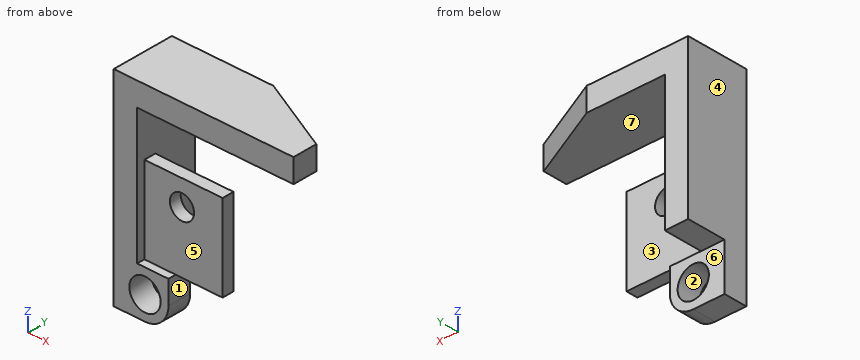
Autodesk Inventor part; units mm, degrees
ref_plane "YZ Plane" through (0, 0, 0) normal (1, 0, 0) x (0, 1, 0)
ref_plane "XZ Plane" through (0, 0, 0) normal (0, 1, 0) x (-1, 0, 0)
ref_plane "XY Plane" through (0, 0, 0) normal (0, 0, 1) x (1, 0, 0)
sketch "Szkic1" plane through (0, 0, 0) normal (0, 1, 0) x (-1, 0, 0)
  line L0 (0, 0) -> (3, 0)
  line L1 (3, 0) -> (3, -22)
  line L2 (3, -22) -> (0, -22)
  line L3 (0, -22) -> (0, 0)
  line L4 (0, 0) -> (-20, 0)
  line L5 (-20, 0) -> (-20, -3)
  line L6 (-20, -3) -> (0, -3)
  line L7 (0, -3) -> (0, 0)
  line L8 (0, -22) -> (-3, -22)
  line L9 (-3, -22) -> (-3, -17)
  line L10 (-3, -17) -> (0, -17)
  line L11 (0, -17) -> (0, -22)
  dimension "d0" = 3
  dimension "d1" = 22
  dimension "d2" = 20
  dimension "d3" = 3
  dimension "d4" = 3
  dimension "d5" = 5
extrude "Wyciągnięcie proste1" add sketch "Szkic1" along normal blind 8
sketch "Szkic2" plane through (20, 0, -3) normal (0, 0, -1) x (-1, 0, 0)
  line L0 (0, 0) -> (0, 8)
  line L1 (0, 0) -> (20, 8)
  line L2 (23, 8) -> (0, 8)
  point P0 (20, 0)
extrude "Wyciągnięcie proste2" cut sketch "Szkic2" against normal blind 3
sketch "Szkic3" plane through (0, 8, 0) normal (0, 1, 0) x (1, 0, 0)
  point P0 (0, 0)
sketch "Szkic4" plane through (3, 0, -17) normal (1, 0, 0) x (0, 0, -1)
  line L0 (5, 0) -> (5, 8)
  line L1 (0, 0) -> (0, 8)
  line L2 (5, 0) -> (0, 0)
  line L3 (0, 0) -> (0, 8)
  line L4 (0, 8) -> (5, 8)
  line L5 (5, 8) -> (5, 0)
  point P0 (-17, 0)
extrude "Wyciągnięcie proste3" cut sketch "Szkic4" against normal blind 3
sketch "Szkic5" plane through (0, 0, -22) normal (0, 0, -1) x (-1, 0, 0)
  line L0 (3, 8) -> (0, 8)
  line L1 (0, 0) -> (3, 0)
  line L2 (3, 0) -> (3, 8)
  line L3 (3, 8) -> (0, 8)
  line L4 (0, 8) -> (0, 0)
extrude "Wyciągnięcie proste4" cut sketch "Szkic5" against normal blind 1.8
sketch "Szkic6" plane through (0, 0, -20.2) normal (0, 0, -1) x (-1, 0, 0)
  line L0 (3, 0) -> (3, 8)
  line L1 (3, 0) -> (-4, 0)
  line L2 (-4, 0) -> (-4, 3)
  line L3 (-4, 3) -> (3, 3)
  line L4 (3, 3) -> (3, 0)
  point P0 (0, 0)
  dimension "d14" = 7
  dimension "d15" = 3
extrude "Wyciągnięcie proste5" add sketch "Szkic6" along normal blind 6
sketch "Szkic7" plane through (0, 3, -20.2) normal (0, 1, 0) x (1, 0, 0)
  circle A0 centre (1, 3) radius 2
  line L0 (-3, 0) -> (-3, 6)
  line L1 (-3, 6) -> (4, 6)
  point P0 (0, -20.2)
  point P1 (-3, 3)
  point P2 (0.5, 6)
  dimension "d18" = 4
  dimension "d19" = 4
  dimension "d20" = 3
extrude "Wyciągnięcie proste6" cut sketch "Szkic7" against normal blind 3
sketch "Szkic8" plane through (-3, 0, 0) normal (0, 0, 1) x (1, 0, 0)
  line L0 (3, 8) -> (13, 8)
  line L1 (23, 0) -> (3, 0)
  line L2 (23, 0) -> (23, 3.137)
  line L3 (13, 8) -> (23, 3.137)
  line L4 (23, 0) -> (3, 8)
  line L5 (3, 8) -> (23, 0)
  dimension "d23" = 10
  dimension "d24" = 3.137
extrude "Wyciągnięcie proste7" add sketch "Szkic8" against normal blind 3
sketch "Szkic9" plane through (0, 0, -3) normal (1, 0, 0) x (0, 0, -1)
  line L0 (0, 0) -> (17.2, 0)
  line L1 (17.2, 0) -> (6.2, 0)
  line L2 (6.2, 0) -> (6.2, 1.5)
  line L3 (6.2, 1.5) -> (17.2, 1.5)
  line L4 (17.2, 1.5) -> (17.2, 0)
  point P0 (-3, 0)
  point P1 (6.2, 0)
  dimension "d27" = 11
  dimension "d35" = 1.5
extrude "Wyciągnięcie proste8" add sketch "Szkic9" along normal blind 10
sketch "Szkic10" plane through (0, 1.5, -9.2) normal (0, 1, 0) x (1, 0, 0)
  circle A0 centre (4.8, 3.2) radius 1.55
  line L0 (0, 0) -> (10, 0)
  line L1 (10, 11) -> (10, 0)
  line L2 (4, 11) -> (10, 11)
  line L3 (0, -6.2) -> (0, 11)
  point P0 (0, -9.2)
  point P1 (5, 0)
  dimension "d30" = 3.1
  dimension "d36" = 7.8
  dimension "d37" = 4.8
extrude "Wyciągnięcie proste9" cut sketch "Szkic10" against normal blind 2
fillet "Fillet1" radius 3 1 edges at (4, 1.5, -26.2)
sketch "Szkic11" plane through (0, 1.5, -9.2) normal (0, 1, 0) x (1, 0, 0)
  circle A0 centre (4.8, 3.2) radius 1.55
  line L0 (0, 0) -> (0, 11)
  line L1 (0, 0) -> (10, 0)
  line L2 (10, 11) -> (10, 0)
  line L3 (4, 11) -> (10, 11)
  line L4 (0, 11) -> (4, 11)
  point P0 (0, -9.2)
extrude "Wyciągnięcie proste10" add sketch "Szkic11" along normal blind 1
sketch "Szkic12" plane through (0, 0, 0) normal (0, -1, 0) x (1, 0, 0)
  line L0 (10, -9.2) -> (10, -20.2)
  line L1 (10, -20.2) -> (4, -20.2)
  line L2 (0, -20.2) -> (4, -20.2)
  line L3 (0, -9.2) -> (0, -20.2)
  line L4 (0, -9.2) -> (10, -9.2)
  circle A0 centre (4.8, -12.4) radius 1.55
  point P0 (0, 0)
extrude "Wyciągnięcie proste11" cut sketch "Szkic12" against normal blind 1
properties part number "lfmw" material "Tworzywo sztuczne PET"
The listing builds one solid part. Answer for the finished solid, in the listing's coordinates (mm). Face numbers are marked on the shaded views. A direction names the side the tool comes from. Round coordinates to 2 decimals unless told otherwise and drop trailing zeros. Loops run counter-clockwise (first coordinate to the right, second up) from the corner with the lowest first, then second, coordinate; pieces in that order, holes last. Notation, with made-up numbers: (33, 26.5) - (82, 26.5) arc R31 ccw to (82, 65.5) - close; hole circle Ø7 at (40, 65). An arc over 180 degrees is marked (long way). Return JSON: item names as keys, results as strings. Group by question number.
1. Which of the six approach directions +Z, -Z, +X, -X, +Y, -Y give full straight-line access (tool end or side, diameter ignored) to the marked faces 5, 6 and 7?
2. The part is cut by section A-A on x = 4.8. Determine the outline of the cut face in (y, z).
3. The part is cut by section D-D on z = -15.75. Determine the outline of the cut face in (x, y).
4. Each of these flat-tipped pins is pushed along its axis until it touches: P1, Ø2, axis at x = 6.5, z = -20, coming from the -Y side; P2, Ø3.5, axis at y = 1, z = -21, coming from the +X side; P3, Ø1, axis at x = 6, z = -14.5, coming from the +Y side; P4, Ø1, axis at x = 13, y = 1, coming from the +Z side. Where does it stop, or does it pass through?
5. The part is cut by section C-C on y = 2. Determine the outline of the cut face in (x, z), then the cut area to 3 significant figures.
6. Consider probe 1 along Z at (x, y) = (1, 1.95); probe 2 along Z at (x, y) = (4.8, 1.9); probe 3 along X at (y, z) = (0.8, -23.2). Determine where each line is inside the solid, lowest interval first.
7. The mould has two halves that part along X. Classify the marked faces 1, 2, 3 and 4: pulls with the +X half, pulls with the -X half, needs draft (parallel to the pull), parting line crosses it, or undercut.
8. The part is cut by section B-B on z = -12.4. Determine the outline of the cut face in (x, y).
Resolved:
{
 "1": {"face 5": "+X, -Y", "face 6": "-Z, +X, -X, +Y", "face 7": "+X, +Y, -Y"},
 "2": {"outline": "(0, -3) - (8, -3) - (8, 0) - (0, 0) - close; (1, -20.2) - (2.5, -20.2) - (2.5, -13.95) - (1, -13.95) - close; (1, -10.85) - (2.5, -10.85) - (2.5, -9.2) - (1, -9.2) - close"},
 "3": {"outline": "(-3, 0) - (0, 0) - (0, 1) - (10, 1) - (10, 2.5) - (0, 2.5) - (0, 8) - (-3, 8) - close"},
 "4": {"P1": "stops at y = 1", "P2": "stops at x = 10", "P3": "stops at y = 2.5", "P4": "stops at z = 0"},
 "5": {"outline": "(-3, -26.2) - (1, -26.2) arc R3 ccw to (4, -23.2) - (4, -20.2) - (10, -20.2) - (10, -9.2) - (0, -9.2) - (0, -3) - (20, -3) - (20, 0) - (-3, 0) - close; hole circle Ø4 at (1, -23.2); hole circle Ø3.1 at (4.8, -12.4)", "area": "251 mm²"},
 "6": {"probe 1": "z = -26.2 to -25.2, -21.2 to -9.2, -3 to 0", "probe 2": "z = -20.2 to -13.95, -10.85 to -9.2, -3 to 0", "probe 3": "x = -3 to -1, 3 to 4"},
 "7": {"face 1": "pulls with the +X half", "face 2": "undercut", "face 3": "needs draft", "face 4": "pulls with the -X half"},
 "8": {"outline": "(-3, 0) - (0, 0) - (0, 1) - (3.25, 1) - (3.25, 2.5) - (0, 2.5) - (0, 8) - (-3, 8) - close; (6.35, 1) - (10, 1) - (10, 2.5) - (6.35, 2.5) - close"}
}
